Drawing for the job (mm, zero at the part's lowest x, y, z). A direction names the side the tool comes from. Give positions to 0.01 mm unless a question says otherwise; leave off trailing zeros. Loops run counter-clockwise (first coordinate to the right, second up) from the corner with the lowest first, then second, coordinate; pieces in that order, holes last. Notation, with made-up numbers: (-3, 16.5) -> (41, 16.5) arc R26 cw to (41, 39.5) -> close; hole circle Ø1 at (-5, 28). An arc over 180 degrees is marked (long way). Use CSV: the item, a comma, the result in double quotes. Start each with the question number.
(1) Flat gauge pins, fed straight in: pin 1 (2 mm diameter, centred on x = 11.5, z = 4, fed in from +Y); pin 2 (1.5 mm diameter, centred on y = 11, z = 1.5, fed in from -X); pin 3 (9 mm diameter, centred on x = 8.5, y = 8.5, fed in from +Z). Where does each tip first touch, or does it go through?
(2) Cut at A-A on x = 8.5. Write the cut outline in (y, z).
(3) Cut at C-C on z = 4.25. Write the cut outline in (x, y).
(4) Pull direction X, two halves, no side cores. Call the marked faces 4, 5, 6 and 7: pulls with the +X half, pulls with the -X half, needs draft (parallel to the pull), parting line crosses it, or undercut.
(5) Cut at D-D on z = 0.6. Write the cut outline in (x, y).
(6) 3-axis set-ups, long thin cutter, end or side, ignore diameter. For the marked faces 1, 2 and 3: which of +Z, -Z, +X, -X, +Y, -Y reach the whole face in a straight line?
(7) Drill centre lines: probe 1 along Z at (x, y) = (5.5, 9.25); probe 2 along X at (y, z) = (8.5, 2.15); probe 3 along Y at (x, z) = (8.5, 0.2). Where is each one in solid material? Low to high.
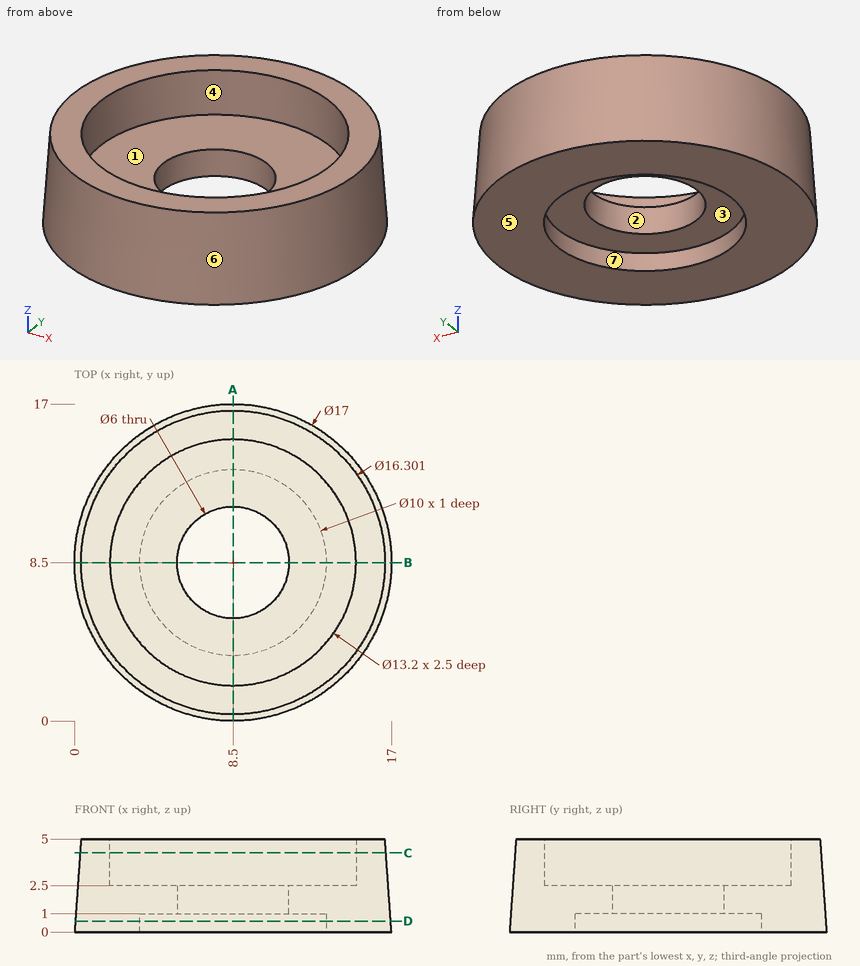
Check result:
1,pin 1,"y = 16.48"
1,pin 2,"x = 0.28"
1,pin 3,"z = 2.5"
2,outline,"(0, 0) -> (3.5, 0) -> (3.5, 1) -> (5.5, 1) -> (5.5, 2.5) -> (1.9, 2.5) -> (1.9, 5) -> (0.35, 5) -> close; (11.5, 1) -> (13.5, 1) -> (13.5, 0) -> (17, 0) -> (16.65, 5) -> (15.1, 5) -> (15.1, 2.5) -> (11.5, 2.5) -> close"
3,outline,"circle Ø16.41 at (8.5, 8.5); hole circle Ø13.2 at (8.5, 8.5)"
4,face 4,"undercut"
4,face 5,"needs draft"
4,face 6,"parting line crosses it"
4,face 7,"undercut"
5,outline,"circle Ø16.92 at (8.5, 8.5); hole circle Ø10 at (8.5, 8.5)"
6,face 1,"+Z"
6,face 2,"+Z, -Z"
6,face 3,"-Z"
7,probe 1,"1 to 2.5"
7,probe 2,"0.15 to 5.5, 11.5 to 16.85"
7,probe 3,"0.01 to 3.5, 13.5 to 16.99"
